Can you work these out from the model? Positions are in its coordinate system, mm. A direction names the side the tool comes from. Coordinates: 2 decimals unless noted, no trailing zeros. Order: outer loops, then holes, each group sorted by start corner. A loop starts at its lowest first (then second) coordinate and runs counter-clockwise, first axis right, second up.
Autodesk Inventor part; units mm, degrees
ref_plane "YZ Plane" through (0, 0, 0) normal (1, 0, 0) x (0, 1, 0)
ref_plane "XZ Plane" through (0, 0, 0) normal (0, 1, 0) x (-1, 0, 0)
ref_plane "XY Plane" through (0, 0, 0) normal (0, 0, 1) x (1, 0, 0)
sketch "Boceto1" plane through (0, 0, 0) normal (0, 0, 1) x (1, 0, 0)
  line L0 (386.3, -100) -> (-386.3, -100)
  line L1 (-386.3, -100) -> (-386.3, 100)
  line L2 (-386.3, 100) -> (386.3, 100)
  line L3 (386.3, 100) -> (386.3, -100)
  line L4 (386.3, -100) -> (-386.3, 100) construction
  line L5 (-386.3, -100) -> (386.3, 100) construction
  point P0 (0, 0)
  dimension "d0" = 772.6
  dimension "d1" = 200
extrude "Placa1" add sketch "Boceto1" along normal blind 2
sketch "Boceto2" plane through (-384.3, -100, 0) normal (-1, 0, 0) x (0, -1, 0)
  line L0 (-200, 0) -> (0, 0)
  line L1 (0, 0) -> (0, 30)
  line L2 (0, 30) -> (-200, 30)
  line L3 (-200, 30) -> (-200, 0)
edge flange "Pestaña1" height 30 angle 90 thickness 2 bend radius 2 thickness toward (-1, 0, 0) relief tear relief width 2 relief depth 1 corner gap 2 corner form 0 edges at (-386.3, 0, 2) (386.3, 0, 2) wall of the first edge with corners at (-384.3, 100, 0) (-384.3, -100, 0) (-384.3, -100, 30) (-384.3, 100, 30)
bend "Doblez1"
corner "Esquina1"
sketch "Boceto3" plane through (386.3, -100, 30) normal (1, 0, 0) x (0, 0, -1)
  circle A0 centre (13, 185) radius 6
  circle A1 centre (13, 15) radius 6
  line L0 (26, 0) -> (0, 0)
  line L1 (0, 200) -> (26, 200)
  point P0 (30, 100)
  point P1 (13, 0)
  point P2 (13, 200)
  dimension "d13" = 12
  dimension "d14" = 12
  dimension "d16" = 15
  dimension "d17" = 15
extrude "Extrusión1" cut sketch "Boceto3" against normal through all
fillet "Redondeo de esquina1" radius 6 4 edges at (385.3, -100, 30) (-385.3, -100, 30) (-385.3, 100, 30) (385.3, 100, 30)
equation "\"d2\" = Thickness"
equation "\"d3\" = BendReliefWidth"
equation "\"d4\" = BendReliefDepth"
equation "\"d5\" = MinimumRemnant"
equation "\"d6\" = TransitionRadius"
equation "\"d9\" = BendRadius"
equation "\"d10\" = CornerReliefSize"
equation "\"d11\" = GapSize"
equation "\"d12\" = JacobiRadiusSize"
equation "\"BendRadius\" = Thickness"
equation "\"BendReliefWidth\" = Thickness"
equation "\"BendReliefDepth\" = 0.5 * Thickness"
equation "\"CornerReliefSize\" = 4 * Thickness"
equation "\"MinimumRemnant\" = 2 * Thickness"
equation "\"TransitionRadius\" = BendRadius"
equation "\"JacobiRadiusSize\" = BendRadius"
equation "\"GapSize\" = Thickness"
properties part number "Conector"
1. Thinking about a two-plate mould opening in Z: for faces 3 (the cylindrical face through (-385.29, -79.05, 17.78)), 4 (the flat face through (-5, 1, 0)), 5 (the flat face through (-5, 1, 2)), which applies, pulls with the +Z half, pulls with the -Z half, needs draft (parallel to the pull), parting line crosses it, or undercut?
Completed:
face 3: undercut
face 4: pulls with the -Z half
face 5: pulls with the +Z half
2. Imagine slicing it at B-B on y = -14. Please give me the cut outline in (x, z), then the cut area to 3 significant figures.
Completed:
outline: (-386.3, 4) arc R4 ccw to (-382.3, 0) - (382.3, 0) arc R4 ccw to (386.3, 4) - (386.3, 30) - (384.3, 30) - (384.3, 4) arc R2 cw to (382.3, 2) - (-382.3, 2) arc R2 cw to (-384.3, 4) - (-384.3, 30) - (-386.3, 30) - close
area: 1,650 mm2
3. On a 3-axis mill with a long thin cutter (end or side, diameter ignored), from which of +Z, -Z, +X, -X, +Y, -Y can I reach the whole of each face in a straight line? I mean faces 1 (the flat face through (-2, 100, 1)), 2 (the flat face through (384.3, 1, 17)). Say none if no direction works.
Completed:
face 1: +Z, -Z, +X, -X, +Y
face 2: +Z, +Y, -Y
4. I'm going to push a flat-ended pin straight in: pin 1 (1 mm diameter, centred on x = -232, y = -67.5, fed in from +Z). Where does the tip first touch, or does it pass through?
Completed:
pin 1: stops at z = 2
5. Please list where these lines run through material, in increasing order: probe 1 along Y at (x, z) = (-385.3, 17); probe 2 along X at (y, z) = (28, 16); probe 3 along X at (y, z) = (85, 3.5).
Completed:
probe 1: y = -100 to -91, -79 to 79, 91 to 100
probe 2: x = -386.3 to -384.3, 384.3 to 386.3
probe 3: x = -386.27 to -384.24, 384.24 to 386.27
6. Imagine slicing it at C-C on x = -176.5. Please give me the cut outline in (y, z).
Completed:
outline: (-100, 0) - (100, 0) - (100, 2) - (-100, 2) - close
7. Imagine slicing it at A-A on z = 17. Please give me the cut outline in (x, y).
Completed:
outline: (-386.3, -100) - (-384.3, -100) - (-384.3, -91) - (-386.3, -91) - close; (-386.3, -79) - (-384.3, -79) - (-384.3, 79) - (-386.3, 79) - close; (-386.3, 91) - (-384.3, 91) - (-384.3, 100) - (-386.3, 100) - close; (384.3, -100) - (386.3, -100) - (386.3, -91) - (384.3, -91) - close; (384.3, -79) - (386.3, -79) - (386.3, 79) - (384.3, 79) - close; (384.3, 91) - (386.3, 91) - (386.3, 100) - (384.3, 100) - close
